The figure shows three views and two pictorial views of one solid part (mm, origin at its lowest corner). Answer the questions. Give positions to 0.01 mm unless a question says otherwise; leave off trailing zeros. Loops run counter-clockwise (first coordinate to the right, second up) from the corner with the lowest first, then second, coordinate; pieces in that order, holes last. Notation, with made-up numbers: M 20.25,-24 L 72.25,-24 A24 cw 72.25,-10 Z; hole C 49,26.25 d11. An arc over 180 degrees is marked long. One line per item, written item: value. Start each with the question number.
Q1. A cutting plane is placed at B-B, the plane y = 2.75. Determine the outline of the cut face in (x, z).
Q2. Consider L1, parallel to X at y = 0.85, z = 2.7; L2, parallel to Y at x = 5.5, z = 2.65; L3, parallel to Y at x = 5.75, z = 0.45. Determine where each line is inside the solid, lowest interval first.
Q3. A cutting plane is placed at A-A, the plane x = 7.25. Determine the outline of the cut face in (y, z).
Q4. A flat-ended cylindrical pin translates along its axis: pin 1 (1.5 mm diameter, centred on y = 3, z = 2.5, fed in from +X). Find the tip coordinate at first contact, or state that the pin passes through.
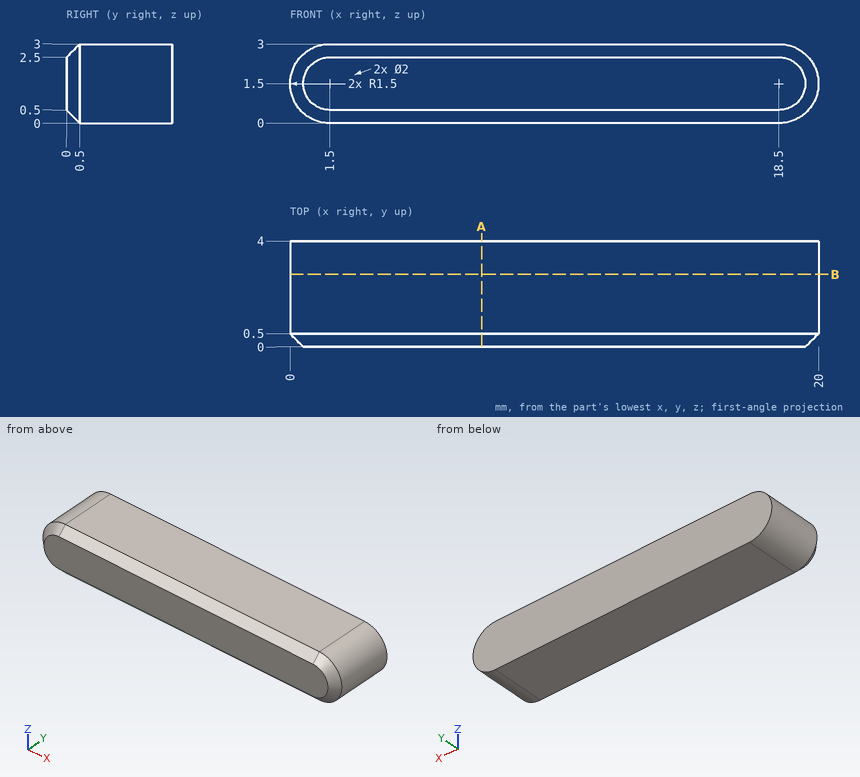
Answer block:
1. outline: M 1.5,0 L 18.5,0 A1.5 ccw 18.5,3 L 1.5,3 A1.5 ccw Z
2. L1: 0.6 to 19.4
2. L2: 0.15 to 4
2. L3: 0.05 to 4
3. outline: M 0,0.5 L 0.5,0 L 4,0 L 4,3 L 0.5,3 L 0,2.5 Z
4. pin 1: x = 19.98
